```python
from build123d import *

# Parameters (mm, degrees)
CROQUIS1_W              = 250
CROQUIS1_H              = 390
CROQUIS1_R              = 44.5
CROQUIS1_W_2            = 77.375
CROQUIS1_H_2            = 294.75
CROQUIS1_H_3            = 151.3
SALIENTE_EXTRUIR1_DEPTH = 12.7
CROQUIS2_W              = 37.2
CROQUIS2_H              = 12.7
CROQUIS2_W_2            = 74.4
CORTAR_EXTRUIR1_DEPTH   = 13.7


with BuildPart() as part:
    # Croquis1 → Saliente-Extruir1 (new body)
    with BuildSketch(Plane.XY):
        Rectangle(CROQUIS1_W, CROQUIS1_H)
        with Locations((62.5, 119.8)):
            Circle(CROQUIS1_R, mode=Mode.SUBTRACT)
        with Locations((-54.5625, 15.875)):
            Rectangle(CROQUIS1_W_2, CROQUIS1_H_2, mode=Mode.SUBTRACT)
        with Locations((54.5625, -55.85)):
            Rectangle(CROQUIS1_W_2, CROQUIS1_H_3, mode=Mode.SUBTRACT)
    extrude(amount=SALIENTE_EXTRUIR1_DEPTH)

    # Croquis2 → Cortar-Extruir1 (cut, through all)
    with BuildSketch(Plane.XY.offset(12.7)):
        with Locations((-106.4, 188.65)):
            Rectangle(CROQUIS2_W, CROQUIS2_H)
        with Locations((0, 188.65)):
            Rectangle(CROQUIS2_W_2, CROQUIS2_H)
        with Locations((106.4, 188.65)):
            Rectangle(CROQUIS2_W, CROQUIS2_H)
        with BuildLine():
            Line((-119.475, 175.95), (-111.475, 175.95))
            ThreePointArc((-111.475, 175.95), (-108.275, 172.75), (-111.475, 169.55))
            Line((-111.475, 169.55), (-119.475, 169.55))
            ThreePointArc((-119.475, 169.55), (-122.675, 172.75), (-119.475, 175.95))
        make_face()
        with BuildLine():
            Line((-4, 175.95), (4, 175.95))
            ThreePointArc((4, 175.95), (7.2, 172.75), (4, 169.55))
            Line((4, 169.55), (-4, 169.55))
            ThreePointArc((-4, 169.55), (-7.2, 172.75), (-4, 175.95))
        make_face()
        with BuildLine():
            Line((111.475, 175.95), (119.475, 175.95))
            ThreePointArc((119.475, 175.95), (122.675, 172.75), (119.475, 169.55))
            Line((119.475, 169.55), (111.475, 169.55))
            ThreePointArc((111.475, 169.55), (108.275, 172.75), (111.475, 175.95))
        make_face()
    cortar_extruir1 = extrude(amount=-CORTAR_EXTRUIR1_DEPTH, mode=Mode.SUBTRACT)

    # Simetría1: Cortar-Extruir1 across plane
    add(cortar_extruir1.mirror(Plane.ZX), mode=Mode.SUBTRACT)


solid = part.part
```
Source: CAD feature listing. Evaluate the final solid. Frame: model axes, mm. A direction names the side the tool comes from. Give positions to 0.01 mm unless a question says otherwise; leave off trailing zeros. Loops run counter-clockwise (first coordinate to the right, second up) from the corner with the lowest first, then second, coordinate; pieces in that order, holes last. Notation, with made-up numbers: M 30.25,9 L 35.25,9 A16 ccw 35.25,31 Z; hole C 25.25,89.25 d11. An arc over 180 degrees is marked long. Put each result on its own line as item: value.
Q1. Section C-C (y = 63). Return the cut outline in (x, z) (3 decimals).
Response values:
outline: M -125,0 L -93.25,0 L -93.25,12.7 L -125,12.7 Z; M -15.875,0 L 125,0 L 125,12.7 L -15.875,12.7 Z
Q2. Section B-B (x = -52.5). Return the cut outline in (y, z).
Response values:
outline: M -195,0 L -131.5,0 L -131.5,12.7 L -195,12.7 Z; M 163.25,0 L 195,0 L 195,12.7 L 163.25,12.7 Z
Q3. Section D-D (x = 62.5). Return the cut outline in (y, z), and give its area (3 significant figures).
Response values:
outline: M -195,0 L -131.5,0 L -131.5,12.7 L -195,12.7 Z; M 19.8,0 L 75.3,0 L 75.3,12.7 L 19.8,12.7 Z; M 164.3,0 L 195,0 L 195,12.7 L 164.3,12.7 Z
area: 1,900 mm²
Q4. Pin query (flat end, axial travel): P1, Ø2.5, axis at x = -116, z = 7, coming from the -Y side; P2, Ø2.5, axis at x = -114, z = 4, coming from the +Y side; P3, Ø4, axis at y = -188, z = 6.5, coming from the -X side. Return the tip coordinate at first contact, or that it passes through.
Response values:
P1: stops at y = -182.3
P2: stops at y = 182.3
P3: stops at x = -87.8
Q5. Mould query, pull axis X, two halves, no side actions, for faces 1 (the flat face through (-87.8, -189, 6)), 2 (the flat face through (106, -182.3, 6)), 3 (the flat face through (-115, -169.55, 6)), 4 (the flat face through (54, 19.8, 6)). Classes: released by +X, released by -X, zero draft, split by the parting line, or undercut.
Response values:
face 1: released by -X
face 2: zero draft
face 3: undercut
face 4: undercut
Q6. Section A-A (y = -116.5). Return the cut outline in (x, z) (3 decimals).
Response values:
outline: M -125,0 L -93.25,0 L -93.25,12.7 L -125,12.7 Z; M -15.875,0 L 15.875,0 L 15.875,12.7 L -15.875,12.7 Z; M 93.25,0 L 125,0 L 125,12.7 L 93.25,12.7 Z
Q7. Reachability of faces 5 (the flat face through (115, 175.95, 6)), 6 (the flat face through (-37.2, 189, 6)), 7 (the flat face through (106, 182.3, 6)) from +Z, -Z, +X, -X, +Y, -Y: full face, straight path, thin tool, end or side. Return the list, or none.
Response values:
face 5: +Z, -Z
face 6: +Z, -Z, +Y
face 7: +Z, -Z, +X, +Y
Q8. Line query: probe 1 along X at (y, z) = (-52.5, 2.5) (3 decimals); probe 2 along Y at (x, z) = (62.5, 4.75); probe 3 along X at (y, z) = (-172.5, 9.5). Output: solid intervals per line, ascending. Write a range as [from, to].
Response values:
probe 1: x = [-125, -93.25], [-15.875, 15.875], [93.25, 125]
probe 2: y = [-195, -131.5], [19.8, 75.3], [164.3, 195]
probe 3: x = [-125, -122.67], [-108.28, -7.19], [7.19, 108.28], [122.67, 125]
